```python
from build123d import *

# Parameters (mm, degrees)
F0_W     = 7.62
F0_H     = 15.875
F1_DEPTH = 4.7625
F2_R     = 2.4511
F3_DEPTH = 1.778
F4_W     = 4.572
F4_H     = 12.827
F4_R     = 1.4986
F5_DEPTH = 8.382


with BuildPart() as f1:
    # F0 (on Top) → F1 (new body, symmetric)
    with BuildSketch(Plane.XY):
        Rectangle(F0_W, F0_H)
    extrude(amount=F1_DEPTH, both=True)

    # F2 (on face) → F3 (join)
    with BuildSketch(Plane.XY.offset(4.7625)):
        with Locations((0, 4.0132)):
            Circle(F2_R)
        with Locations((0, -4.0132)):
            Circle(F2_R)
    extrude(amount=F3_DEPTH)

    # F4 (on face) → F5 (cut)
    with BuildSketch(Plane(origin=(0, 0, -4.7625), x_dir=(1, 0, 0), z_dir=(0, 0, -1))):
        Rectangle(F4_W, F4_H)
        Circle(F4_R, mode=Mode.SUBTRACT)
    extrude(amount=-F5_DEPTH, mode=Mode.SUBTRACT)


solid = f1.part
```
Model file for the job. Use its own axes, mm. A direction names the side the tool comes from. Round coordinates to 2 decimals unless told otherwise and drop trailing zeros. Loops run counter-clockwise (first coordinate to the right, second up) from the corner with the lowest first, then second, coordinate; pieces in that order, holes last. Notation, with made-up numbers: M 40.5,64 L 66.5,64 A27 cw 66.5,97 Z; hole C -16.75,52 d3. An arc over 180 degrees is marked long. Put each result on its own line as item: value. Start each with the question number.
Item 1: Cut at D-D (y = 2.5). List the corners of the cut face in (x, z).
Item 2: Mould opens along X. For faces 1 (the face through (-3.81, 0, 0)), 2 (the face through (0, 4, 6.54)), 3 (the face through (-2.286, 0, -1)), 4 (the face through (2.286, 0, -1)) say: released by +X, released by -X, zero draft, split by the parting line, or undercut.
Item 3: 3-axis set-ups, long thin cutter, end or side, ignore diameter. For faces 5 (the face through (0, 0, 4.762)), 6 (the face through (0, 6.414, -1)), 7 (the face through (0, 7.938, 0)): which of +Z, -Z, +X, -X, +Y, -Y reach the whole face in a straight line?
Item 4: Cut at B-B (x = 0). List the corners of the cut face in (y, z).
Item 5: Cut at A-A (z = 2.75). List the corners of the cut face in (x, y), then the cut area to 3 significant figures.
Item 6: Cut at C-C (y = 0). List the corners of the cut face in (x, z), then the cut area to 3 significant figures.
Item 7: Drill centre lines: line 1 along Y through (x, z) = (0, 3.5); line 2 along X through (y, z) = (-2, -3.5); line 3 along Y through (x, z) = (1.25, -2.75). Where is each one in solid material? Low to high.
Answer block:
1. outline: M -3.81,-4.76 L -2.29,-4.76 L -2.29,3.62 L 2.29,3.62 L 2.29,-4.76 L 3.81,-4.76 L 3.81,4.76 L 1.93,4.76 L 1.93,6.54 L -1.93,6.54 L -1.93,4.76 L -3.81,4.76 Z
2. face 1: released by -X
2. face 2: zero draft
2. face 3: undercut
2. face 4: undercut
3. face 5: +Z
3. face 6: -Z
3. face 7: +Z, -Z, +X, -X, +Y
4. outline: M -7.94,-4.76 L -6.41,-4.76 L -6.41,3.62 L -1.5,3.62 L -1.5,-4.76 L 1.5,-4.76 L 1.5,3.62 L 6.41,3.62 L 6.41,-4.76 L 7.94,-4.76 L 7.94,4.76 L 6.46,4.76 L 6.46,6.54 L 1.56,6.54 L 1.56,4.76 L -1.56,4.76 L -1.56,6.54 L -6.46,6.54 L -6.46,4.76 L -7.94,4.76 Z
5. outline: M -3.81,-7.94 L 3.81,-7.94 L 3.81,7.94 L -3.81,7.94 Z; C 0,0 d3; hole M -2.29,-6.41 L 2.29,-6.41 L 2.29,6.41 L -2.29,6.41 Z
5. area: 69.4 mm2
6. outline: M -3.81,-4.76 L -2.29,-4.76 L -2.29,3.62 L -1.5,3.62 L -1.5,-4.76 L 1.5,-4.76 L 1.5,3.62 L 2.29,3.62 L 2.29,-4.76 L 3.81,-4.76 L 3.81,4.76 L -3.81,4.76 Z
6. area: 59.4 mm2
7. line 1: -7.94 to -6.41, -1.5 to 1.5, 6.41 to 7.94
7. line 2: -3.81 to -2.29, 2.29 to 3.81
7. line 3: -7.94 to -6.41, -0.83 to 0.83, 6.41 to 7.94
